```python
from build123d import *

# Parameters (mm, degrees)
ESQUISSE1_W             = 57.9
ESQUISSE1_H             = 86
BOSS_EXTRU_1_DEPTH      = 7
ESQUISSE3_R             = 2.1
ESQUISSE3_R_2           = 5.1
ENL_V_MAT_EXTRU_2_DEPTH = 53.30776711
ESQUISSE4_R             = 3.75
ENL_V_MAT_EXTRU_3_DEPTH = 4.3
ESQUISSE6_R             = 3.75
ENL_V_MAT_EXTRU_5_DEPTH = 4.3
ESQUISSE7_W             = 28
ESQUISSE7_H             = 29
ENL_V_MAT_EXTRU_6_DEPTH = 4
ESQUISSE9_R             = 1.975
ESQUISSE9_W             = 14
ESQUISSE9_H             = 5
ENL_V_MAT_EXTRU_7_DEPTH = 52.991369476
ESQUISSE10_R            = 2.35
ENL_V_MAT_EXTRU_8_DEPTH = 53.30776711


with BuildPart() as part:
    # Esquisse1 → Boss.-Extru.1 (new body)
    with BuildSketch(Plane.XY):
        Rectangle(ESQUISSE1_W, ESQUISSE1_H)
    extrude(amount=BOSS_EXTRU_1_DEPTH)

    # Esquisse3 → Enlèv. mat.-Extru.2 (cut, through all)
    with BuildSketch(Plane(origin=(0, 0, 0), x_dir=(-1, 0, 0), z_dir=(0, 0, -1))):
        with Locations((23.95, 38)):
            Circle(ESQUISSE3_R)
        with Locations((-23.960388264, 38.019803714)):
            Circle(ESQUISSE3_R)
        with Locations((23.95, -38)):
            Circle(ESQUISSE3_R)
        with Locations((-23.95, -38)):
            Circle(ESQUISSE3_R)
        with Locations((1.229278893, -29.411147051)):
            Circle(ESQUISSE3_R_2)
    extrude(amount=-ENL_V_MAT_EXTRU_2_DEPTH, mode=Mode.SUBTRACT)

    # Esquisse4 → Enlèv. mat.-Extru.3 (cut)
    with BuildSketch(Plane(origin=(0, 0, 0), x_dir=(-1, 0, 0), z_dir=(0, 0, -1))):
        with Locations((23.95, -38)):
            Circle(ESQUISSE4_R)
        with Locations((-23.95, -38)):
            Circle(ESQUISSE4_R)
        with Locations((23.95, 38)):
            Circle(ESQUISSE4_R)
    extrude(amount=-ENL_V_MAT_EXTRU_3_DEPTH, mode=Mode.SUBTRACT)

    # Esquisse6 → Enlèv. mat.-Extru.5 (cut)
    with BuildSketch(Plane(origin=(0, 0, 0), x_dir=(-1, 0, 0), z_dir=(0, 0, -1))):
        with Locations((-23.95, 38)):
            Circle(ESQUISSE6_R)
    extrude(amount=-ENL_V_MAT_EXTRU_5_DEPTH, mode=Mode.SUBTRACT)

    # Esquisse7 → Enlèv. mat.-Extru.6 (cut)
    with BuildSketch(Plane(origin=(0, 0, 0), x_dir=(-1, 0, 0), z_dir=(0, 0, -1))):
        with Locations((0, -8)):
            Rectangle(ESQUISSE7_W, ESQUISSE7_H)
    extrude(amount=-ENL_V_MAT_EXTRU_6_DEPTH, mode=Mode.SUBTRACT)

    # Esquisse9 → Enlèv. mat.-Extru.7 (cut, through all)
    with BuildSketch(Plane(origin=(0, 0, 4), x_dir=(-1, 0, 0), z_dir=(0, 0, -1))):
        with Locations((11.78, -19.99)):
            Circle(ESQUISSE9_R)
        with Locations((-11.78, -19.99)):
            Circle(ESQUISSE9_R)
        with Locations((-11.78, 3.99)):
            Circle(ESQUISSE9_R)
        with Locations((11.78, 3.99)):
            Circle(ESQUISSE9_R)
        with Locations((0, 3.01)):
            Rectangle(ESQUISSE9_W, ESQUISSE9_H)
    extrude(amount=-ENL_V_MAT_EXTRU_7_DEPTH, mode=Mode.SUBTRACT)

    # Esquisse10 → Enlèv. mat.-Extru.8 (cut, through all)
    with BuildSketch(Plane(origin=(0, 0, 0), x_dir=(-1, 0, 0), z_dir=(0, 0, -1))):
        with Locations((0, 15)):
            Circle(ESQUISSE10_R)
    extrude(amount=-ENL_V_MAT_EXTRU_8_DEPTH, mode=Mode.SUBTRACT)


solid = part.part
```
Source: CAD feature listing. Evaluate the final solid. Frame: model axes, mm. A direction names the side the tool comes from. Give positions to 0.01 mm unless a question says otherwise; leave off trailing zeros. Order: outer loops, then holes, each group sorted by start corner. A loop starts at its lowest first (then second) coordinate and runs counter-clockwise, first axis right, second up.
(1) Contact query for flat-ended pins moving along their axis: P1, Ø14, axis at x = 4, y = -14.5, coming from the -Z side; P2, Ø5.5, axis at x = -23.95, y = 38, coming from the -Z side; P3, Ø3, axis at x = 11.78, y = -19.99, coming from the +Z side. Output: stop coordinate, or through.
(2) Material intervals for line 1 along X through (y, z) = (1, 0.75); line 2 along Y through (x, z) = (-23.95, 2.95); line 3 along Y through (x, z) = (11.78, 5.65) (3 decimals), sorted ascending.
(3) Section query D-D (x = 0). Return the cut outline in (y, z), plus the area to 3 significant figures.
(4) Pull-direction query (Y, two-part tool) for faces 3 (the face through (-26, -40, 4.3)), 4 (the face through (0, -43, 3)), 5 (the face through (0, 10, 0)); classes: +Y half, -Y half, draft (parallel to the pull), parting line (faces both ways), or undercut.
(5) Section query C-C (x = -11.78). Return the cut outline in (y, z) (3 decimals).
(6) Access query for faces 1 (the face through (0, 5.51, 5)), 2 (the face through (26.926, -40.282, 2.12)). Directions: +Z, -Z, +X, -X, +Y, -Y. A direction counts if a zero-diameter tool reaches every point of the face in a straight line with its end or side. Return the directions, or none.
(7) Section query B-B (y = -19.99). Return the cut outline in (x, z) (3 decimals), plus the area to 3 significant figures.
(8) Section query A-A (y = 15). Return the cut outline in (x, z), plus the area to 3 significant figures.
Outcome:
1. P1: stops at z = 4
1. P2: stops at z = 4.3
1. P3: passes through
2. line 1: x = -28.95 to -14, 14 to 28.95
2. line 2: y = -43 to -41.75, -34.25 to 34.25, 41.75 to 43
2. line 3: y = -43 to -21.965, -18.015 to 2.015, 5.965 to 43
3. outline: (-43, 0) - (-34.36, 0) - (-34.36, 7) - (-43, 7) - close; (-24.46, 0) - (-22.5, 0) - (-22.5, 4) - (0.51, 4) - (0.51, 7) - (-24.46, 7) - close; (5.51, 4) - (6.5, 4) - (6.5, 0) - (12.65, 0) - (12.65, 7) - (5.51, 7) - close; (17.35, 0) - (43, 0) - (43, 7) - (17.35, 7) - close
3. area: 369 mm2
4. face 3: undercut
4. face 4: -Y half
4. face 5: draft
5. outline: (-43, 0) - (-22.5, 0) - (-22.5, 4) - (-21.965, 4) - (-21.965, 7) - (-43, 7) - close; (-18.015, 4) - (2.015, 4) - (2.015, 7) - (-18.015, 7) - close; (5.965, 4) - (6.5, 4) - (6.5, 0) - (43, 0) - (43, 7) - (5.965, 7) - close
6. face 1: +Z, -Z
6. face 2: -Z
7. outline: (-28.95, 0) - (-14, 0) - (-14, 4) - (-13.755, 4) - (-13.755, 7) - (-28.95, 7) - close; (-9.805, 4) - (9.805, 4) - (9.805, 7) - (-9.805, 7) - close; (13.755, 4) - (14, 4) - (14, 0) - (28.95, 0) - (28.95, 7) - (13.755, 7) - close
7. area: 270 mm2
8. outline: (-28.95, 0) - (-2.35, 0) - (-2.35, 7) - (-28.95, 7) - close; (2.35, 0) - (28.95, 0) - (28.95, 7) - (2.35, 7) - close
8. area: 372 mm2
